Can you work these out from the drawing? Everything is in mm from the part's minimum corner. A direction names the side the tool comes from. Coordinates: 2 decimals unless noted, no trailing zeros. Write each loop counter-clockwise with the first axis right and the second up, starting at its lowest first coordinate (ties: lowest second). Pieces come first, ordered by that corner, then holes.
(1) Imagine slicing it at D-D, the plane x = 9. List the corners of the cut face in (y, z) for me, plus the area to 3 significant figures.
(2) Imagine slicing it at B-B, the plane x = 29. List the corners of the cut face in (y, z) for me.
(3) Imagine slicing it at A-A, the plane y = 29. List the corners of the cut face in (x, z) for me, plus the area to 3 significant figures.
(4) Thinking about a two-plate mould opening in X: for the marked faces 3, 4 and 5, which applies, released by +X, released by -X, zero draft, split by the parting line, or undercut?
(5) Please list where these lines run through material, in increasing order: probe 1 along Y at (x, z) = (29, 4.75); probe 2 along X at (y, z) = (39.5, 4) (1 decimal); probe 3 along Y at (x, z) = (51, 5) (1 decimal).
(6) For pin 1 Ø6.5 at (x, y) = (49.78, 41) entering from +Z; pin 2 Ø10 at (y, z) = (24, 17) entering from -X; pin 3 Ø2 at (x, z) = (18, 3.5) entering from +Y, each with a flat end and sliding along its axis, tell me the tip position at first contact or that it passes through.
(7) Imagine slicing it at C-C, the plane z = 20.25. List the corners of the cut face in (x, y) for me, plus the area to 3 significant figures.
(8) Which directions (+Z, -Z, +X, -X, +Y, -Y) give clear straight access to the entire face, cutting with the end or side of a thin tool? Please do the marked faces 1 and 2.
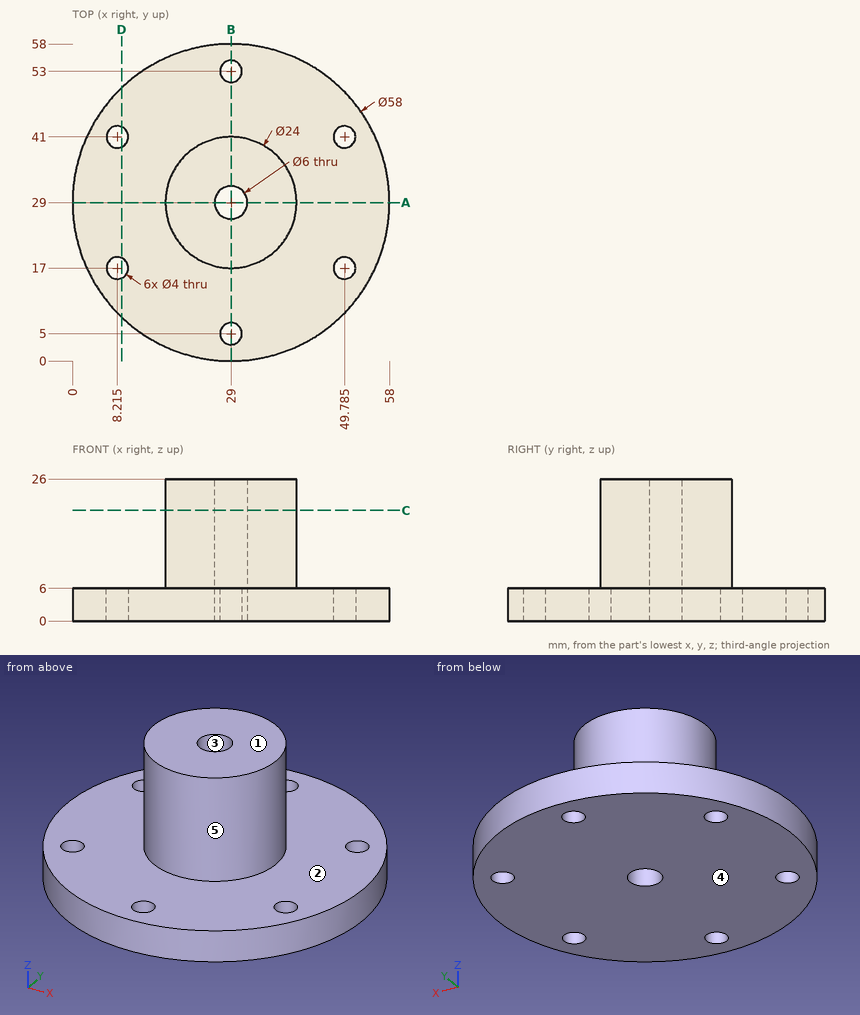
Recorded:
1. outline: (8, 0) - (15.16, 0) - (15.16, 6) - (8, 6) - close; (18.84, 0) - (39.16, 0) - (39.16, 6) - (18.84, 6) - close; (42.84, 0) - (50, 0) - (50, 6) - (42.84, 6) - close
1. area: 208 mm2
2. outline: (0, 0) - (3, 0) - (3, 6) - (0, 6) - close; (7, 0) - (26, 0) - (26, 26) - (17, 26) - (17, 6) - (7, 6) - close; (32, 0) - (51, 0) - (51, 6) - (41, 6) - (41, 26) - (32, 26) - close; (55, 0) - (58, 0) - (58, 6) - (55, 6) - close
3. outline: (0, 0) - (26, 0) - (26, 26) - (17, 26) - (17, 6) - (0, 6) - close; (32, 0) - (58, 0) - (58, 6) - (41, 6) - (41, 26) - (32, 26) - close
3. area: 672 mm2
4. face 3: undercut
4. face 4: zero draft
4. face 5: split by the parting line
5. probe 1: y = 0 to 3, 7 to 26, 32 to 51, 55 to 58
5. probe 2: x = 2 to 6.9, 9.5 to 48.5, 51.1 to 56
5. probe 3: y = 10.1 to 15.4, 18.6 to 39.4, 42.6 to 47.9
6. pin 1: stops at z = 6
6. pin 2: stops at x = 17
6. pin 3: stops at y = 56.22
7. outline: circle Ø24 at (29, 29); hole circle Ø6 at (29, 29)
7. area: 424 mm2
8. face 1: +Z, +X, -X, +Y, -Y
8. face 2: +Z
